The listing builds one solid part. Answer for the finished solid, in the listing's coordinates (mm). A direction names the side the tool comes from. Coordinates: 2 decimals unless noted, no trailing zeros. Order: outer loops, then holes, each group sorted by start corner. A loop starts at its lowest first (then second) coordinate and runs counter-clockwise, first axis right, second up.
```python
from build123d import *

# Parameters (mm, degrees)
F1_DEPTH = 9.525


with BuildPart() as f1:
    # F0 (on Top) → F1 (new body)
    with BuildSketch(Plane.XY):
        with BuildLine():
            ThreePointArc((66.675, 31.75), (62.955256, 40.730256), (53.975, 44.45))
            Line((53.975, 44.45), (42.480119, 44.45))
            ThreePointArc((42.480119, 44.45), (38.146553, 43.687764), (34.333175, 41.492551))
            ThreePointArc((34.333175, 41.492551), (0, 29.029153), (-34.333175, 41.492551))
            ThreePointArc((-34.333175, 41.492551), (-38.146553, 43.687764), (-42.480119, 44.45))
            Line((-42.480119, 44.45), (-53.975, 44.45))
            ThreePointArc((-53.975, 44.45), (-62.955256, 40.730256), (-66.675, 31.75))
            Line((-66.675, 31.75), (-66.675, 25.355166))
            ThreePointArc((-66.675, 25.355166), (-66.054129, 21.432839), (-64.25222, 17.894017))
            ThreePointArc((-64.25222, 17.894017), (-58.441686, 0), (-64.25222, -17.894017))
            ThreePointArc((-64.25222, -17.894017), (-66.054129, -21.432839), (-66.675, -25.355166))
            Line((-66.675, -25.355166), (-66.675, -31.75))
            ThreePointArc((-66.675, -31.75), (-62.955256, -40.730256), (-53.975, -44.45))
            Line((-53.975, -44.45), (-42.480119, -44.45))
            ThreePointArc((-42.480119, -44.45), (-38.146553, -43.687764), (-34.333175, -41.492551))
            ThreePointArc((-34.333175, -41.492551), (0, -29.029153), (34.333175, -41.492551))
            ThreePointArc((34.333175, -41.492551), (38.146553, -43.687764), (42.480119, -44.45))
            Line((42.480119, -44.45), (53.975, -44.45))
            ThreePointArc((53.975, -44.45), (62.955256, -40.730256), (66.675, -31.75))
            Line((66.675, -31.75), (66.675, -25.355166))
            ThreePointArc((66.675, -25.355166), (66.054129, -21.432839), (64.25222, -17.894017))
            ThreePointArc((64.25222, -17.894017), (58.441686, 0), (64.25222, 17.894017))
            ThreePointArc((64.25222, 17.894017), (66.054129, 21.432839), (66.675, 25.355166))
            Line((66.675, 25.355166), (66.675, 31.75))
        make_face()
        with BuildLine():
            ThreePointArc((-53.925, -37.75), (-59.925, -31.75), (-53.925, -25.75))
            Line((-53.925, -25.75), (-50.8, -25.75))
            ThreePointArc((-50.8, -25.75), (-44.8, -31.75), (-50.8, -37.75))
            Line((-50.8, -37.75), (-53.925, -37.75))
        make_face(mode=Mode.SUBTRACT)
        with BuildLine():
            ThreePointArc((53.925, -25.75), (59.925, -31.75), (53.925, -37.75))
            Line((53.925, -37.75), (50.75, -37.75))
            ThreePointArc((50.75, -37.75), (44.75, -31.75), (50.75, -25.75))
            Line((50.75, -25.75), (53.925, -25.75))
        make_face(mode=Mode.SUBTRACT)
        with BuildLine():
            ThreePointArc((-53.925, 25.75), (-59.925, 31.75), (-53.925, 37.75))
            Line((-53.925, 37.75), (-50.8, 37.75))
            ThreePointArc((-50.8, 37.75), (-44.8, 31.75), (-50.8, 25.75))
            Line((-50.8, 25.75), (-53.925, 25.75))
        make_face(mode=Mode.SUBTRACT)
        with BuildLine():
            ThreePointArc((53.925, 37.75), (59.925, 31.75), (53.925, 25.75))
            Line((53.925, 25.75), (50.75, 25.75))
            ThreePointArc((50.75, 25.75), (44.75, 31.75), (50.75, 37.75))
            Line((50.75, 37.75), (53.925, 37.75))
        make_face(mode=Mode.SUBTRACT)
    extrude(amount=F1_DEPTH)


solid = f1.part
```
1) Each of these flat-tipped pins is pushed along its axis until it touches: P1, Ø4, axis at y = -3.5, z = 8, coming from the -X side; P2, Ø4, axis at x = 18.5, z = 2.5, coming from the +Y side; P3, Ø3, axis at y = -5.5, z = 2, coming from the +X side. Where does it stop, or does it pass through?
2) A cutting plane is placed at D-D, the plane y = -12.5. Write down the section's boundary in (x, z) (3 decimals).
3) A cutting plane is placed at C-C, the plane x = 46.5. Write down the section's boundary in (y, z) (3 decimals), plus the area to 3 significant figures.
4) Straight lines are drawn through the part: probe 1 along Y at (x, z) = (-57, 7.25); probe 2 along X at (y, z) = (29, 8) (3 decimals); probe 3 along X at (y, z) = (28, 1.75) (3 decimals). For each, find the intervals that lie inside material, in ascending order.
5) A cutting plane is placed at B-B, the plane z = 5.5. Count the separate pieces of the cut face and the enclosed holes in it, plus the area to 3 significant figures.
6) The mould has two halves that part along X. Classify faces 1 (the cylindrical face through (66.071, -21.486, 4.696)), 2 (the cylindrical face through (-66.071, 21.486, 4.696)), 3 (the cylindrical face through (59.924, 31.882, 4.696)): released by +X, released by -X, zero draft, split by the parting line, or undercut.
7) A cutting plane is placed at A-A, the plane x = -47.5. Write down the section's boundary in (y, z) (3 decimals).
8) For faces 4 (the cylindrical face through (-38.088, 43.666, 4.696)), 5 (the flat face through (52, -25.75, 5)), 6 (the cylindrical face through (-66.037, -21.38, 4.696)), 7 (the cylindrical face through (-38.205, -43.709, 4.696)), determine the directions among +Z, -Z, +X, -X, +Y, -Y from which every point of the face is accessible in a straight line to the end or side of a thin tool.
Working result:
1. P1: stops at x = -58.94
1. P2: stops at y = 33.11
1. P3: stops at x = 59.26
2. outline: (-61.125, 0) - (61.125, 0) - (61.125, 9.525) - (-61.125, 9.525) - close
3. outline: (-44.45, 0) - (-35.985, 0) - (-35.985, 9.525) - (-44.45, 9.525) - close; (-27.515, 0) - (27.515, 0) - (27.515, 9.525) - (-27.515, 9.525) - close; (35.985, 0) - (44.45, 0) - (44.45, 9.525) - (35.985, 9.525) - close
3. area: 685 mm2
4. probe 1: y = -44.08 to -36.9, -26.6 to 26.6, 36.9 to 44.08
4. probe 2: x = -66.675 to -59.258, -45.467 to 45.417, 59.258 to 66.675
4. probe 3: x = -66.675 to -58.609, -46.116 to 46.066, 58.609 to 66.675
5. separate pieces: 1
5. enclosed holes: 4
5. area: 9,030 mm2
6. face 1: released by +X
6. face 2: released by -X
6. face 3: undercut
7. outline: (-44.45, 0) - (-36.761, 0) - (-36.761, 9.525) - (-44.45, 9.525) - close; (-26.739, 0) - (26.739, 0) - (26.739, 9.525) - (-26.739, 9.525) - close; (36.761, 0) - (44.45, 0) - (44.45, 9.525) - (36.761, 9.525) - close
8. face 4: +Z, -Z, +Y
8. face 5: +Z, -Z
8. face 6: +Z, -Z, -X
8. face 7: +Z, -Z, -Y
